```python
from build123d import *

# Parameters (mm, degrees)
F0_W      = 35
F0_H      = 37
F1_DEPTH  = 4.5
F2_R      = 1.5
F3_DEPTH  = 10
F4_W      = 35
F4_H      = 10
F5_DEPTH  = 10
F6_R      = 3
F7_DEPTH  = 6
F8_W      = 35
F8_H      = 4.5
F9_DEPTH  = 2
F10_W     = 8
F10_H     = 25
F10_W_2   = 13.5
F11_DEPTH = 14.501
F12_W     = 15
F12_H     = 5
F13_DEPTH = 4.501
F14_R     = 3
F15_R     = 1.5
F16_DEPTH = 21.501


with BuildPart() as f1:
    # F0 (on Front) → F1 (new body)
    with BuildSketch(Plane.XZ):
        with Locations((0, -1.5)):
            Rectangle(F0_W, F0_H)
    extrude(amount=F1_DEPTH)

    # F2 (on face) → F3 (cut)
    with BuildSketch(Plane.XZ.offset(4.5)):
        with Locations((12.5, -15)):
            Circle(F2_R)
        with Locations((-12.5, -15)):
            Circle(F2_R)
    extrude(amount=-F3_DEPTH, mode=Mode.SUBTRACT)

    # F4 (on face) → F5 (join)
    with BuildSketch(Plane.XZ.offset(4.5)):
        with Locations((0, 12)):
            Rectangle(F4_W, F4_H)
    extrude(amount=F5_DEPTH)

    # F6 (on face) → F7 (cut)
    with BuildSketch(Plane(origin=(0, 0, 7), x_dir=(1, 0, 0), z_dir=(0, 0, -1))):
        with Locations((-2.75, 9.5)):
            Circle(F6_R)
    extrude(amount=-F7_DEPTH, mode=Mode.SUBTRACT)

    # F8 (on face) → F9 (cut)
    with BuildSketch(Plane(origin=(0, 0, -20), x_dir=(1, 0, 0), z_dir=(0, 0, -1))):
        with Locations((0, 2.25)):
            Rectangle(F8_W, F8_H)
    extrude(amount=-F9_DEPTH, mode=Mode.SUBTRACT)

    # F10 (on face) → F11 (cut, through all)
    with BuildSketch(Plane.XZ.offset(14.5)):
        with Locations((-13.5, 4.5)):
            Rectangle(F10_W, F10_H)
        with Locations((10.75, 4.5)):
            Rectangle(F10_W_2, F10_H)
    extrude(amount=-F11_DEPTH, mode=Mode.SUBTRACT)

    # F12 (on face) → F13 (cut, through all)
    with BuildSketch(Plane.XZ.offset(4.5)):
        with Locations((-2, -15.5)):
            Rectangle(F12_W, F12_H)
    extrude(amount=-F13_DEPTH, mode=Mode.SUBTRACT)

    # F14
    f14_edges = [f1.edges().sort_by_distance(p)[0] for p in [
        (5.5, -2.25, -13),
        (-9.5, -2.25, -13),
    ]]
    fillet(f14_edges, radius=F14_R)

    # F15 (on face) → F16 (cut, through all)
    with BuildSketch(Plane.YZ.offset(4)):
        with Locations((-9.5, 10)):
            Circle(F15_R)
    extrude(amount=-F16_DEPTH, mode=Mode.SUBTRACT)


solid = f1.part
```
Verification items for the finished model (mm, model axes). A direction names the side the tool comes from. Round coordinates to 2 decimals unless told otherwise and drop trailing zeros. Write each loop counter-clockwise with the first axis right and the second up, starting at its lowest first coordinate (ties: lowest second). Pieces come first, ordered by that corner, then holes. Notation, with made-up numbers: (60.25, 5.5) -> (111.25, 5.5) arc R14 cw to (111.25, 16.5) -> close; hole circle Ø9 at (13, 39). An arc over 180 degrees is marked (long way). Write each question's results on one line, items separated by ' | '. Start each with the question number.
1. Draft check along X on faces 1 (the flat face through (-14, -2, -18)), 2 (the flat face through (-9.5, -4, 7)), 3 (the flat face through (-3, -10, 13)). Enter one of: +X half, -X half, draft (parallel to the pull), parting line (faces both ways), or undercut.
2. Cross-section at B-B (y = -9.5). Enter the section's corners in (x, z), then the cut area to 3 significant figures.
3. Cross-section at A-A (z = 10). Enter the section's corners in (x, y), then the cut area to 3 significant figures.
4. Set-up check for faces 4 (the flat face through (4, -4, 7)), 5 (the flat face through (-9.5, -2, -17)), 6 (the flat face through (-14, -2, -8)), 7 (the flat face through (-6, -9, 7)): record each of +Z, -Z, +X, -X, +Y, -Y from which the full face is reachable in a straight line by a thin tool's end or side.
5. Cross-section at C-C (x = -12.5). Enter the section's corners in (y, z), then the cut area to 3 significant figures.
6. Cross-section at D-D (y = -3.25). Enter the section's corners in (x, z).
7. Depth check by flat-ended pin: P1, Ø2, axis at x = -0.5, y = -2.5, coming from the -Z side; P2, Ø1.3, axis at x = 8, y = -1.5, coming from the +Z side; P3, Ø5, axis at x = -4, y = -8.5, coming from the -Z side; P4, Ø2.5, axis at x = 12.5, z = -15, coming from the +Y side. Enter the tip coordinate at first touch or a pass-through.
8. Material ranges on probe 1 along Z at (x, y) = (2.65, -9.5); probe 2 along Y at (x, z) = (-2.75, 10.25); probe 3 along X at (y, z) = (-4.25, -17), recorded low to high. Write a range as from..to.
Solutions:
1) face 1: draft | face 2: -X half | face 3: undercut
2) outline: (-9.5, 7) -> (-5.75, 7) -> (-5.75, 8.5) -> (-9.5, 8.5) -> close; (-9.5, 11.5) -> (-5.75, 11.5) -> (-5.75, 13) -> (0.25, 13) -> (0.25, 11.5) -> (4, 11.5) -> (4, 17) -> (-9.5, 17) -> close; (0.25, 7) -> (4, 7) -> (4, 8.5) -> (0.25, 8.5) -> close | area: 76.5 mm2
3) outline: (-9.5, -14.5) -> (4, -14.5) -> (4, -11) -> (-0.15, -11) arc R3 cw to (-5.35, -11) -> (-9.5, -11) -> close; (-9.5, -8) -> (-5.35, -8) arc R3 cw to (-0.15, -8) -> (4, -8) -> (4, 0) -> (-9.5, 0) -> close | area: 144 mm2
4) face 4: +Z, +X, +Y, -Y | face 5: -Z, +Y, -Y | face 6: +Z, -X, +Y, -Y | face 7: -Z, +X, -X, -Y
5) outline: (-4.5, -18) -> (0, -18) -> (0, -16.5) -> (-4.5, -16.5) -> close; (-4.5, -13.5) -> (0, -13.5) -> (0, -8) -> (-4.5, -8) -> close | area: 31.5 mm2
6) outline: (-17.5, -18) -> (-9.5, -18) -> (-9.5, -16) arc R3 cw to (-6.5, -13) -> (2.5, -13) arc R3 cw to (5.5, -16) -> (5.5, -18) -> (17.5, -18) -> (17.5, -8) -> (4, -8) -> (4, 17) -> (-9.5, 17) -> (-9.5, -8) -> (-17.5, -8) -> close; hole circle Ø3 at (-12.5, -15); hole circle Ø3 at (12.5, -15)
7) P1: stops at z = -13 | P2: stops at z = -8 | P3: stops at z = 7 | P4: passes through
8) probe 1: z = 7..8.5, 11.5..17 | probe 2: y = -14.5..-12.5, -6.5..0 | probe 3: x = -17.5..-9.5, 5.5..17.5
